Here's how the part is built. I have some questions about the finished solid (model axes, mm). Face numbers are marked on the shaded views. A direction names the side the tool comes from. Round coordinates to 2 decimals unless told otherwise and drop trailing zeros. Order: outer loops, then holes, each group sorted by start corner. A loop starts at its lowest first (then second) coordinate and runs counter-clockwise, first axis right, second up. Notation, with made-up numbers: (-33.75, 46.25) - (-19.75, 46.25) arc R34 ccw to (-19.75, 76.25) - close; hole circle Ø4 at (32.25, 2.25). An arc over 180 degrees is marked (long way). Answer as a JSON object with one key per item and string values.
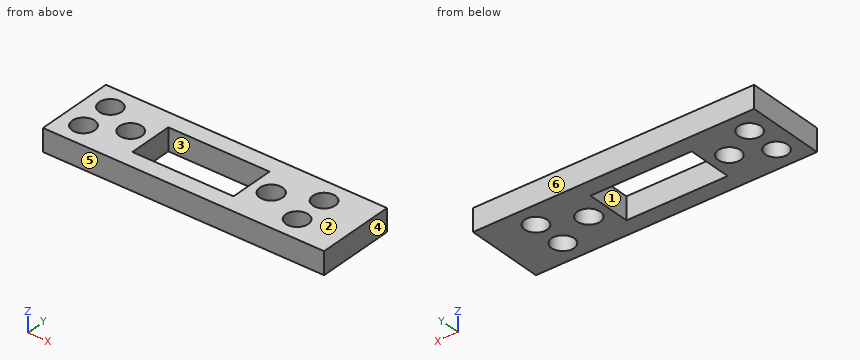
```python
from build123d import *

# Parameters (mm, degrees)
CYLINDER005_R     = 1
CYLINDER005_DEPTH = 2
CYLINDER004_R     = 1
CYLINDER004_DEPTH = 2
CYLINDER003_R     = 1
CYLINDER003_DEPTH = 2
CYLINDER002_R     = 1
CYLINDER002_DEPTH = 2
CYLINDER001_R     = 1
CYLINDER001_DEPTH = 2
CYLINDER_R        = 1.02
CYLINDER_DEPTH    = 2
BOX001_W          = 9
BOX001_H          = 4
BOX001_DEPTH      = 2
BOX_W             = 25
BOX_H             = 7
BOX_DEPTH         = 2


with BuildPart() as cylinder005:
    # Cylinder005 → Cylinder005 (new body)
    with BuildSketch(Plane(origin=(16, 5, 0), x_dir=(1, 0, 0), z_dir=(0, 0, 1))):
        Circle(CYLINDER005_R)
    extrude(amount=CYLINDER005_DEPTH)


with BuildPart() as cylinder004:
    # Cylinder004 → Cylinder004 (new body)
    with BuildSketch(Plane(origin=(16, 2, 0), x_dir=(1, 0, 0), z_dir=(0, 0, 1))):
        Circle(CYLINDER004_R)
    extrude(amount=CYLINDER004_DEPTH)


with BuildPart() as cylinder003:
    # Cylinder003 → Cylinder003 (new body)
    with BuildSketch(Plane(origin=(-3, 2, 0), x_dir=(1, 0, 0), z_dir=(0, 0, 1))):
        Circle(CYLINDER003_R)
    extrude(amount=CYLINDER003_DEPTH)


with BuildPart() as cylinder002:
    # Cylinder002 → Cylinder002 (new body)
    with BuildSketch(Plane(origin=(-3, 5, 0), x_dir=(1, 0, 0), z_dir=(0, 0, 1))):
        Circle(CYLINDER002_R)
    extrude(amount=CYLINDER002_DEPTH)


with BuildPart() as cylinder001:
    # Cylinder001 → Cylinder001 (new body)
    with BuildSketch(Plane(origin=(0, 3.5, 0), x_dir=(1, 0, 0), z_dir=(0, 0, 1))):
        Circle(CYLINDER001_R)
    extrude(amount=CYLINDER001_DEPTH)


with BuildPart() as cylinder:
    # Cylinder → Cylinder (new body)
    with BuildSketch(Plane(origin=(12.5, 3.5, 0), x_dir=(1, 0, 0), z_dir=(0, 0, 1))):
        Circle(CYLINDER_R)
    extrude(amount=CYLINDER_DEPTH)


with BuildPart() as cube001:
    # Box001 → Box001 (new body)
    with BuildSketch(Plane(origin=(1.75, 1.5, 0), x_dir=(1, 0, 0), z_dir=(0, 0, 1))):
        with Locations((4.5, 2)):
            Rectangle(BOX001_W, BOX001_H)
    extrude(amount=BOX001_DEPTH)


with BuildPart() as cut006:
    # Box → Box (new body)
    with BuildSketch(Plane(origin=(-5, 0, 0), x_dir=(1, 0, 0), z_dir=(0, 0, 1))):
        with Locations((12.5, 3.5)):
            Rectangle(BOX_W, BOX_H)
    extrude(amount=BOX_DEPTH)

    # Cut: cut Cube001
    add(cube001.part, mode=Mode.SUBTRACT)

    # Cut001: cut Cylinder
    add(cylinder.part, mode=Mode.SUBTRACT)

    # Cut002: cut Cylinder001
    add(cylinder001.part, mode=Mode.SUBTRACT)

    # Cut003: cut Cylinder002
    add(cylinder002.part, mode=Mode.SUBTRACT)

    # Cut004: cut Cylinder003
    add(cylinder003.part, mode=Mode.SUBTRACT)

    # Cut005: cut Cylinder004
    add(cylinder004.part, mode=Mode.SUBTRACT)

    # Cut006: cut Cylinder005
    add(cylinder005.part, mode=Mode.SUBTRACT)


solid = cut006.part
```
1. For P1, Ø1.8, axis at x = 16, y = 2, coming from the -Z side; P2, Ø2.5, axis at x = 0, y = 3.5, coming from the +Z side, each with a flat end and sliding along its axis, tell me the tip position at first contact or that it passes through.
Responses:
{"P1": "through", "P2": "z = 2"}
2. For the marked faces 1 and 2, which set-ups out of +Z, -Z, +X, -X, +Y, -Y let a thin tool reach every point of the face, with its end or its side?
Responses:
{"face 1": "+Z, -Z", "face 2": "+Z, +X, -X, +Y, -Y"}
3. Imagine slicing it at B-B (y = 5). List the corners of the cut face in (x, z) for me, plus the area to 3 significant figures.
Responses:
{"outline": "(-5, 0) - (-4, 0) - (-4, 2) - (-5, 2) - close; (-2, 0) - (1.75, 0) - (1.75, 2) - (-2, 2) - close; (10.75, 0) - (15, 0) - (15, 2) - (10.75, 2) - close; (17, 0) - (20, 0) - (20, 2) - (17, 2) - close", "area": "24.0 mm2"}
4. Imagine slicing it at C-C (z = 0.75). List the corners of the cut face in (x, y) for me.
Responses:
{"outline": "(-5, 0) - (20, 0) - (20, 7) - (-5, 7) - close; hole circle Ø2 at (-3, 2); hole circle Ø2 at (-3, 5); hole circle Ø2 at (0, 3.5); hole (1.75, 1.5) - (10.75, 1.5) - (10.75, 5.5) - (1.75, 5.5) - close; hole circle Ø2.04 at (12.5, 3.5); hole circle Ø2 at (16, 2); hole circle Ø2 at (16, 5)"}
5. If I drill on L1, parallel to Y at x = -3, z = 0.8; L2, parallel to Y at x = 12.5, z = 1.45; L3, parallel to Y at x = 10, z = 0.4, over which ranges is the centre line in solid material (lowest first)? Write a range as [from, to].
Responses:
{"L1": "[0, 1], [3, 4], [6, 7]", "L2": "[0, 2.48], [4.52, 7]", "L3": "[0, 1.5], [5.5, 7]"}
6. Imagine slicing it at A-A (x = 0). List the corners of the cut face in (y, z) for me.
Responses:
{"outline": "(0, 0) - (2.5, 0) - (2.5, 2) - (0, 2) - close; (4.5, 0) - (7, 0) - (7, 2) - (4.5, 2) - close"}
7. Thinking about a two-plate mould opening in Y: for the marked faces 3, 4, 5 and 6, which applies, pulls with the +Y half, pulls with the -Y half, needs draft (parallel to the pull), parting line crosses it, or undercut?
Responses:
{"face 3": "undercut", "face 4": "needs draft", "face 5": "pulls with the -Y half", "face 6": "pulls with the +Y half"}
8. Imagine slicing it at D-D (x = 16). List the corners of the cut face in (y, z) for me.
Responses:
{"outline": "(0, 0) - (1, 0) - (1, 2) - (0, 2) - close; (3, 0) - (4, 0) - (4, 2) - (3, 2) - close; (6, 0) - (7, 0) - (7, 2) - (6, 2) - close"}
